from build123d import *

# Parameters (mm, degrees)
SKETCH_1_R      = 15.35
SKETCH_1_R_2    = 2.5
EXTRUDE_1_DEPTH = 15
EXTRUDE_START   = 5
EXTRUDE_2_DEPTH = 5
FILLET_1_R      = 1.5


with BuildPart() as part:
    # Sketch 1 → Extrude 1 (new body)
    with BuildSketch(Plane.XY):
        Circle(SKETCH_1_R)
        Circle(SKETCH_1_R_2, mode=Mode.SUBTRACT)
    extrude(amount=EXTRUDE_1_DEPTH)

    # Sketch 1_3 → Extrude 2 (add)
    with BuildSketch(Plane.XY.offset(EXTRUDE_START)):
        with BuildLine():
            Line((0, 20.35), (0, 15.35))
            ThreePointArc((0, 15.35), (2.863230175, 15.080597235), (5.625957141, 14.281845337))
            Line((5.625957141, 14.281845337), (4, 20.35))
            Line((4, 20.35), (0, 20.35))
        make_face()
        with BuildLine():
            Line((-4, 20.35), (-5.625957141, 14.281845337))
            ThreePointArc((-5.625957141, 14.281845337), (-2.863230175, 15.080597235), (0, 15.35))
            Line((0, 15.35), (0, 20.35))
            Line((0, 20.35), (-4, 20.35))
        make_face()
        with BuildLine():
            Line((11.561195872, 17.218050122), (6.120637241, 14.076942131))
            ThreePointArc((6.120637241, 14.076942131), (10.854089091, 10.854089091), (14.076942131, 6.120637241))
            Line((14.076942131, 6.120637241), (17.218050122, 11.561195872))
            Line((17.218050122, 11.561195872), (11.561195872, 17.218050122))
        make_face()
        with BuildLine():
            Line((20.35, 4), (14.281845337, 5.625957141))
            ThreePointArc((14.281845337, 5.625957141), (15.080597235, 2.863230175), (15.35, 0))
            ThreePointArc((15.35, 0), (15.080597235, -2.863230175), (14.281845337, -5.625957141))
            Line((14.281845337, -5.625957141), (20.35, -4))
            Line((20.35, -4), (20.35, 4))
        make_face()
        with BuildLine():
            Line((17.218050122, -11.561195872), (14.076942131, -6.120637241))
            ThreePointArc((14.076942131, -6.120637241), (10.854089091, -10.854089091), (6.120637241, -14.076942131))
            Line((6.120637241, -14.076942131), (11.561195872, -17.218050122))
            Line((11.561195872, -17.218050122), (17.218050122, -11.561195872))
        make_face()
        with BuildLine():
            ThreePointArc((5.625957141, -14.281845337), (0, -15.35), (-5.625957141, -14.281845337))
            Line((-5.625957141, -14.281845337), (-4, -20.35))
            Line((-4, -20.35), (4, -20.35))
            Line((4, -20.35), (5.625957141, -14.281845337))
        make_face()
        with BuildLine():
            ThreePointArc((-6.120637241, -14.076942131), (-10.854089091, -10.854089091), (-14.076942131, -6.120637241))
            Line((-14.076942131, -6.120637241), (-17.218050122, -11.561195872))
            Line((-17.218050122, -11.561195872), (-11.561195872, -17.218050122))
            Line((-11.561195872, -17.218050122), (-6.120637241, -14.076942131))
        make_face()
        with BuildLine():
            ThreePointArc((-14.281845337, -5.625957141), (-15.35, 0), (-14.281845337, 5.625957141))
            Line((-14.281845337, 5.625957141), (-20.35, 4))
            Line((-20.35, 4), (-20.35, -4))
            Line((-20.35, -4), (-14.281845337, -5.625957141))
        make_face()
        with BuildLine():
            ThreePointArc((-14.076942131, 6.120637241), (-10.854089091, 10.854089091), (-6.120637241, 14.076942131))
            Line((-6.120637241, 14.076942131), (-11.561195872, 17.218050122))
            Line((-11.561195872, 17.218050122), (-17.218050122, 11.561195872))
            Line((-17.218050122, 11.561195872), (-14.076942131, 6.120637241))
        make_face()
    extrude(amount=EXTRUDE_2_DEPTH)

    # Fillet 1
    fillet_1_edges = [part.edges().sort_by_distance(p)[0] for p in [
        (4, 20.35, 7.5),
        (-4, 20.35, 7.5),
        (17.218050122, 11.561195872, 7.5),
        (11.561195872, 17.218050122, 7.5),
        (20.35, -4, 7.5),
        (20.35, 4, 7.5),
        (11.561195872, -17.218050122, 7.5),
        (17.218050122, -11.561195872, 7.5),
        (-4, -20.35, 7.5),
        (4, -20.35, 7.5),
        (-17.218050122, -11.561195872, 7.5),
        (-11.561195872, -17.218050122, 7.5),
        (-20.35, 4, 7.5),
        (-20.35, -4, 7.5),
        (-11.561195872, 17.218050122, 7.5),
        (-17.218050122, 11.561195872, 7.5),
    ]]
    fillet(fillet_1_edges, radius=FILLET_1_R)


solid = part.part
Geometry check sheet. Reference: the model listing, model coordinates, mm. A direction names the side the tool comes from. Give positions to 0.01 mm unless a question says otherwise; leave off trailing zeros. Loops run counter-clockwise (first coordinate to the right, second up) from the corner with the lowest first, then second, coordinate; pieces in that order, holes last. Notation, with made-up numbers: M 48.5,-32 L 94.5,-32 A11 cw 94.5,-21 Z; hole C 79,11.5 d9. An arc over 180 degrees is marked long. Answer as a JSON object with one key per item and string values. Group by question number.
Item 1: Mould release check, pull along X, two halves, no side actions. Record for faces 5 (the flat face through (-8.31, 15.34, 7.46)), 6 (the flat face through (-15.34, -8.31, 7.46)), 7 (the cylindrical face through (-11.5, 16.83, 7.54)), 8 (the cylindrical face through (20.032, 3.773, 7.535)): pulls with the +X half, pulls with the -X half, needs draft (parallel to the pull), parting line crosses it, or undercut.
Item 2: Sectioned sample at C-C on x = -7.5. Record the boundary of the cut face in (y, z).
Item 3: Sectioned sample at D-D on z = 12.25. Record the boundary of the cut face in (x, y), plus the area to 3 significant figures.
Item 4: Gauge pin test, flat ends, axial feed: pin 1 (3 mm diameter, centred on x = -1.5, y = -18.5, fed in from -Z); pin 2 (1.8 mm diameter, centred on x = 0, y = -17.5, fed in from +Z); pin 3 (5 mm diameter, centred on x = 6, z = 11, fed in from +Y). Record the tip position at first contact, or that the pin passes through.
Item 5: Material ranges on L1, parallel to Y at x = 0, z = 7; L2, parallel to Y at x = 0, z = 11.5; L3, parallel to Z at x = 11.5, y = -15, recorded low to high.
Item 6: Access from +Z, -Z, +X, -X, +Y, -Y to the whole of each face (thin tool, end or side, straight path). Record for faces 1 (the flat face through (15.378, -8.374, 7.465)), 2 (the flat face through (13, -13, 10)), 3 (the flat face through (-13, -13, 5)), 4 (the flat face through (-15.378, 8.374, 7.465)).
Item 7: Sectioned sample at A-A on y = 0. Record the boundary of the cut face in (x, z).
Findings below:
{
 "1": {"face 5": "undercut", "face 6": "pulls with the -X half", "face 7": "undercut", "face 8": "pulls with the +X half"},
 "2": {"outline": "M -14.87,5 L -13.39,5 L -13.39,0 L 13.39,0 L 13.39,5 L 14.87,5 L 14.87,10 L 13.39,10 L 13.39,15 L -13.39,15 L -13.39,10 L -14.87,10 Z"},
 "3": {"outline": "C 0,0 d30.7; hole C 0,0 d5", "area": "721 mm2"},
 "4": {"pin 1": "z = 5", "pin 2": "z = 10", "pin 3": "y = 20.08"},
 "5": {"L1": "-20.35 to -2.5, 2.5 to 20.35", "L2": "-15.35 to -2.5, 2.5 to 15.35", "L3": "5 to 10"},
 "6": {"face 1": "+Z, -Z, +X", "face 2": "+Z, +X, -Y", "face 3": "-Z, -X, -Y", "face 4": "+Z, -Z, -X"},
 "7": {"outline": "M -20.35,5 L -15.35,5 L -15.35,0 L -2.5,0 L -2.5,15 L -15.35,15 L -15.35,10 L -20.35,10 Z; M 2.5,0 L 15.35,0 L 15.35,5 L 20.35,5 L 20.35,10 L 15.35,10 L 15.35,15 L 2.5,15 Z"}
}
